from build123d import *

# Parameters (mm, degrees)
SKETCH1_W           = 200
SKETCH1_H           = 200
BOSS_EXTRUDE1_DEPTH = 10
SKETCH2_R           = 19.385831102
BOSS_EXTRUDE2_DEPTH = 20
FILLET1_R           = 10


with BuildPart() as part:
    # Sketch1 → Boss-Extrude1 (new body)
    with BuildSketch(Plane.XY):
        with Locations((44.53125, 36.71875)):
            Rectangle(SKETCH1_W, SKETCH1_H)
    extrude(amount=BOSS_EXTRUDE1_DEPTH)

    # Sketch2 → Boss-Extrude2 (add)
    with BuildSketch(Plane.XY.offset(10)):
        with Locations((43.320392106, 105.737649961)):
            Circle(SKETCH2_R)
    extrude(amount=BOSS_EXTRUDE2_DEPTH)

    # Fillet1
    fillet1_edges = [part.edges().sort_by_distance(p)[0] for p in [
        (23.934561004, 105.737649961, 30),
    ]]
    fillet(fillet1_edges, radius=FILLET1_R)


solid = part.part
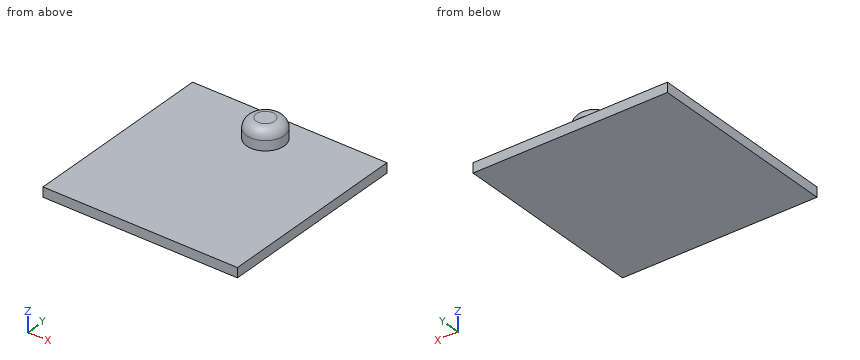
Build history of the part. All positions in model axes, mm. Round coordinates to 2 decimals unless told otherwise and drop trailing zeros. Order: outer loops, then holes, each group sorted by start corner. A loop starts at its lowest first (then second) coordinate and runs counter-clockwise, first axis right, second up. Notation, with made-up numbers: M -25,-5.5 L 24,-5.5 A15 cw 24,6.5 Z; hole C -3,-12 d3. An arc over 180 degrees is marked long. Use CSV: the item, a comma, the result in double quotes. Start each with the question number.
(1) Drill centre lines: probe 1 along Z at (x, y) = (-44.5, -1); probe 2 along X at (y, z) = (113.5, 11); probe 3 along Y at (x, z) = (55.5, 26.5). Where is each one in solid material? Low to high.
(2) Flat gauge pins, fed straight in: P1, Ø4, axis at x = 82.5, y = 82, coming from the +Z side; P2, Ø6, axis at y = 63, z = 15.5, coming from the -X side; P3, Ø1.5, axis at y = 113, z = 19.5, coming from the -X side; P4, Ø12, axis at y = 89.5, z = 20.5, coming from the -X side. Where does each tip first touch, or does it go through?
(3) Cut at A-A on x = 110. List the corners of the cut face in (y, z), then the cut area to 3 significant figures.
(4) Cut at C-C on z = 14. List the corners of the cut face in (x, y), then the cut area to 3 significant figures.
(5) Cut at B-B on y = -29. List the corners of the cut face in (x, z).
Findings:
1,probe 1,"z = 0 to 10"
1,probe 2,"x = 25.56 to 61.08"
1,probe 3,"y = 93.9 to 117.58"
2,P1,"stops at z = 10"
2,P2,"passes through"
2,P3,"stops at x = 25.06"
2,P4,"stops at x = 26.87"
3,outline,"M -63.28,0 L 136.72,0 L 136.72,10 L -63.28,10 Z"
3,area,"2,000 mm^2"
4,outline,"C 43.32,105.74 d38.77"
4,area,"1,180 mm^2"
5,outline,"M -55.47,0 L 144.53,0 L 144.53,10 L -55.47,10 Z"
